Autodesk Inventor part; units mm, degrees
ref_plane "YZ Plane" through (0, 0, 0) normal (1, 0, 0) x (0, 1, 0)
ref_plane "XZ Plane" through (0, 0, 0) normal (0, 1, 0) x (-1, 0, 0)
ref_plane "XY Plane" through (0, 0, 0) normal (0, 0, 1) x (1, 0, 0)
sketch "Sketch1" plane through (0, 0, 0) normal (0, 0, 1) x (1, 0, 0)
  line L0 (-25.4863, -2.2875) -> (-25.4863, -4.4623)
  line L1 (-25.4863, -9.0343) -> (-25.4863, -11.209)
  line L2 (-25.4863, -11.209) -> (-23.8988, -11.209)
  line L3 (-23.8988, -11.209) -> (-23.8988, -2.2875)
  line L4 (-23.8988, -2.2875) -> (-25.4863, -2.2875)
  line L5 (-19.1363, -1.7348) -> (-19.1363, -11.209)
  arc A0 (-27.0661, -8.8868) -> (-27.0661, -4.6098) centre (-27.8739, -6.7483) ccw
  line L6 (-27.0392, -9.0343) -> (-25.4863, -9.0343)
  line L7 (-25.4863, -4.4623) -> (-27.0392, -4.4623)
  arc A1 (-27.0392, -4.4623) -> (-27.0661, -4.6098) centre (-27.0392, -4.5385) ccw
  arc A2 (-27.0661, -8.8868) -> (-27.0392, -9.0343) centre (-27.0392, -8.9581) ccw
  dimension "d0" = 2.1747
  dimension "d2" = 2.1747
  dimension "d3" = 1.5875
  dimension "d7" = 4.572
  dimension "d8" = 0.0762
  dimension "d16" = 4.7625
  dimension "d20" = 3.1404
  dimension "d21" = 3.9751
revolve "Revolution1" add sketch "Sketch1" angle 360 about axis through (-19.1363, -1.7348, 0) along (0, -1, 0)
chamfer "Chamfer1" distance 0.254 angle 45 1 edges at (-12.7863, -2.2875, 0)
chamfer "Chamfer2" distance 0.254 angle 45 3 edges at (-14.3738, -2.2875, 0) (-12.7863, -11.209, 0) (-14.3738, -11.209, 0)
properties part number "Inner Ring 1764"
The listing builds one solid part. Answer for the finished solid, in the listing's coordinates (mm). A direction names the side the tool comes from. Give positions to 0.01 mm unless a question says otherwise; leave off trailing zeros. Loops run counter-clockwise (first coordinate to the right, second up) from the corner with the lowest first, then second, coordinate; pieces in that order, holes last. Notation, with made-up numbers: (-9.5, 51.5) - (49.5, 51.5) arc R16 cw to (49.5, 80.5) - close; hole circle Ø7 at (71, -40). An arc over 180 degrees is marked (long way). Answer as a JSON object with one key per item and string values.
1. For faces 4 (the flat face through (-19.1, -4.462, -6.5)), 5 (the flat face through (-14, -2.288, 1)), 6 (the cylindrical face through (-25.193, -10.008, -1.907)), determine the directions among +Z, -Z, +X, -X, +Y, -Y from which every point of the face is accessible in a straight line to the end or side of a thin tool.
Determined:
{"face 4": "+Y", "face 5": "+Z, -Z, +X, -X, +Y", "face 6": "-Y"}
2. A cutting plane is placed at B-B (y = -8.25). Write down the section's boundary in (x, z) (1 decimal), then the cut area to 3 significant figures.
Determined:
{"outline": "circle Ø14 at (-19.1, 0); hole circle Ø9.5 at (-19.1, 0)", "area": "83.3 mm²"}
3. Flat-ended cylindrical pins translate along their axes: pin 1 Ø1.5 at (x, y) = (-24, -4.5) entering from -Z; pin 2 Ø1.5 at (y, z) = (-10, -4) entering from -X; pin 3 Ø1 at (y, z) = (-5, -1.5) entering from -X. Find the tip coordinate at first contact, or state that the pin passes through.
Determined:
{"pin 1": "z = -6.84", "pin 2": "x = -24.59", "pin 3": "x = -27.01"}
4. For a pull along Z with two mould halves and no side action, classify faces 1 (the cylindrical face through (-14.38, -6.69, 0.21)), 2 (the flat face through (-19.1, -9.034, -6.5)), 3 (the cylindrical face through (-25.193, -3.515, -1.907)) as pulls with the +Z half, pulls with the -Z half, needs draft (parallel to the pull), parting line crosses it, or undercut.
Determined:
{"face 1": "undercut", "face 2": "needs draft", "face 3": "parting line crosses it"}
5. Find the intervals of material crossed by L1, parallel to X at y = -4.25, z = 0; L2, parallel to Z at x = -16.75, y = -8.75; L3, parallel to Z at x = -20.75, y = -10, in increasing order. Write a range as [from, to].
Determined:
{"L1": "[-25.49, -23.9], [-14.37, -12.79]", "L2": "[-7.25, -4.12], [4.12, 7.25]", "L3": "[-6.14, -4.48], [4.48, 6.14]"}
